Autodesk Inventor part; units mm, degrees
ref_plane "YZ Plane" through (0, 0, 0) normal (1, 0, 0) x (0, 1, 0)
ref_plane "XZ Plane" through (0, 0, 0) normal (0, 1, 0) x (-1, 0, 0)
ref_plane "XY Plane" through (0, 0, 0) normal (0, 0, 1) x (1, 0, 0)
sketch "Sketch8" plane through (0, 0, 0) normal (0, 1, 0) x (-1, 0, 0)
  line L0 (37.5, 50) -> (-37.5, 50)
  line L1 (-37.5, 50) -> (-37.5, -50)
  line L2 (-37.5, -50) -> (37.5, -50)
  line L3 (37.5, -50) -> (37.5, 50)
  point P0 (0, 0)
  point P1 (37.5, 0)
  point P2 (0, 50)
  dimension "d42" = 100
  dimension "d43" = 75
extrude "Extrusion5" add sketch "Sketch8" along normal blind 12
sketch "Sketch9" plane through (0, 12, 0) normal (0, 1, 0) x (1, 0, 0)
  line L0 (-37.5, 50) -> (-37.5, -50)
  line L1 (-37.5, -50) -> (37.5, -50)
  point P0 (0, 0)
  point P1 (-33.5, -46)
  point P2 (-33.5, 36)
  point P3 (33.5, 36)
  point P4 (33.5, -46)
  dimension "d46" = 67
  dimension "d47" = 82
  dimension "d48" = 4
  dimension "d49" = 4
hole "Hole3" at (-33.5, 12, 46) at (-33.5, 12, -36) at (33.5, 12, -36) at (33.5, 12, 46) direction (0, -1, 0) diameter 3.2 end through all
sketch "Sketch10" plane through (0, 12, 0) normal (0, 1, 0) x (1, 0, 0)
  line L0 (37.5, 50) -> (-37.5, 50)
  point P0 (0, 0)
  point P1 (-31, -36)
  point P2 (-31, 46)
  point P3 (31, 46)
  point P4 (31, -36)
  dimension "d57" = 62
  dimension "d58" = 82
  dimension "d59" = 4
  dimension "d60" = 31
hole "Hole4" at (-31, 12, 36) at (-31, 12, -46) at (31, 12, -46) at (31, 12, 36) direction (0, -1, 0) diameter 3.2 end through all
sketch "Sketch11" plane through (37.5, 0, 50) normal (1, 0, 0) x (0, 0, -1)
  line L0 (10, 8.5) -> (80, 8.5)
  line L1 (80, 8.5) -> (80, 0)
  line L2 (80, 0) -> (10, 0)
  line L3 (10, 0) -> (10, 8.5)
  line L4 (0, 0) -> (0, 12)
  line L5 (0, 0) -> (100, 0)
  point P0 (50, 0)
  point P1 (45, 0)
  dimension "d69" = 8.5
  dimension "d70" = 70
  dimension "d71" = 45
extrude "Extrusion6" cut sketch "Sketch11" against normal through all
sketch "Sketch12" plane through (-37.5, 0, 50) normal (0, 0, 1) x (1, 0, 0)
  line L0 (6.5, 8.5) -> (68.5, 8.5)
  line L1 (68.5, 8.5) -> (68.5, 0)
  line L2 (68.5, 0) -> (6.5, 0)
  line L3 (6.5, 0) -> (6.5, 8.5)
  line L4 (0, 0) -> (75, 0)
  point P0 (37.5, 0)
  point P1 (37.5, 0)
  dimension "d74" = 8.5
  dimension "d75" = 62
extrude "Extrusion7" cut sketch "Sketch12" against normal through all
sketch "Sketch13" plane through (37.5, 0, -50) normal (1, 0, 0) x (0, 0, -1)
  line L0 (0, 0) -> (0, 12)
  line L1 (0, 0) -> (-10, 0)
  line L2 (-10, 0) -> (-10, 8.5)
  line L3 (-10, 8.5) -> (0, 8.5)
  line L4 (0, 8.5) -> (0, 0)
  line L5 (-20, 8.5) -> (-20, 0)
  line L6 (-90, 8.5) -> (-20, 8.5)
  point P0 (-50, 0)
  dimension "d78" = 10
extrude "Extrusion8" cut sketch "Sketch13" against normal through all
fillet "Fillet1" radius 4 6 edges at (-37.5, 4.25, -40) (-37.5, 10.25, -50) (-37.5, 6, 50) (37.5, 6, 50) (37.5, 4.25, -40) (37.5, 10.25, -50)
sketch "Sketch14" plane through (0, 12, 0) normal (0, 1, 0) x (1, 0, 0)
  line L0 (-23.5, -44) -> (23.5, -44)
  line L1 (27.5, -40) -> (27.5, 40)
  line L2 (23.5, 44) -> (-23.5, 44)
  line L3 (-27.5, 40) -> (-27.5, -40)
  line L4 (-33.5, -50) -> (33.5, -50)
  line L5 (33.5, 50) -> (-33.5, 50)
  line L6 (-37.5, 46) -> (-37.5, -46)
  line L7 (37.5, -46) -> (37.5, 46)
  arc A0 (-27.5, -40) -> (-23.5, -44) centre (-23.5, -40) ccw
  arc A1 (23.5, -44) -> (27.5, -40) centre (23.5, -40) ccw
  arc A2 (27.5, 40) -> (23.5, 44) centre (23.5, 40) ccw
  arc A3 (-23.5, 44) -> (-27.5, 40) centre (-23.5, 40) ccw
  point P0 (0, 0)
  dimension "d82" = 6
  dimension "d83" = 6
  dimension "d84" = 10
  dimension "d85" = 10
  dimension "d86" = 4
extrude "Extrusion9" cut sketch "Sketch14" against normal through all
sketch "Sketch15" plane through (0, 12, 0) normal (0, 1, 0) x (1, 0, 0)
  circle A0 centre (-31, 46) radius 1.6
  circle A1 centre (-31, 46) radius 3
  circle A2 centre (-31, -36) radius 1.6
  circle A3 centre (-31, -36) radius 3
  circle A4 centre (31, -36) radius 1.6
  circle A5 centre (31, -36) radius 3
  circle A6 centre (31, 46) radius 1.6
  circle A7 centre (31, 46) radius 3
  point P0 (0, 0)
  dimension "d89" = 6
  dimension "d90" = 6
  dimension "d91" = 6
  dimension "d92" = 6
extrude "Extrusion10" add sketch "Sketch15" along normal blind 5
sketch "Sketch16" plane through (37.5, 8.5, -30) normal (0, -1, 0) x (1, 0, 0)
  circle A0 centre (-6.5, 66) radius 1.6
  circle A1 centre (-6.5, 66) radius 3
  line L0 (-6.5, 63) -> (-9.0981, 64.5)
  line L1 (-9.0981, 64.5) -> (-9.0981, 67.5)
  line L2 (-9.0981, 67.5) -> (-6.5, 69)
  line L3 (-6.5, 69) -> (-3.9019, 67.5)
  line L4 (-3.9019, 67.5) -> (-3.9019, 64.5)
  line L5 (-3.9019, 64.5) -> (-6.5, 63)
  circle A2 centre (-68.5, -16) radius 1.6
  circle A3 centre (-68.5, -16) radius 3
  line L6 (-68.5, -13) -> (-65.9019, -14.5)
  line L7 (-65.9019, -14.5) -> (-65.9019, -17.5)
  line L8 (-65.9019, -17.5) -> (-68.5, -19)
  line L9 (-68.5, -19) -> (-71.0981, -17.5)
  line L10 (-71.0981, -17.5) -> (-71.0981, -14.5)
  line L11 (-71.0981, -14.5) -> (-68.5, -13)
  circle A4 centre (-68.5, 66) radius 1.6
  circle A5 centre (-68.5, 66) radius 3
  line L12 (-68.5, 63) -> (-71.0981, 64.5)
  line L13 (-71.0981, 64.5) -> (-71.0981, 67.5)
  line L14 (-71.0981, 67.5) -> (-68.5, 69)
  line L15 (-68.5, 69) -> (-65.9019, 67.5)
  line L16 (-65.9019, 67.5) -> (-65.9019, 64.5)
  line L17 (-65.9019, 64.5) -> (-68.5, 63)
  circle A6 centre (-6.5, -16) radius 3
  line L18 (-6.5, -19) -> (-9.0981, -17.5)
  line L19 (-9.0981, -17.5) -> (-9.0981, -14.5)
  line L20 (-9.0981, -14.5) -> (-6.5, -13)
  line L21 (-6.5, -13) -> (-3.9019, -14.5)
  line L22 (-3.9019, -14.5) -> (-3.9019, -17.5)
  line L23 (-3.9019, -17.5) -> (-6.5, -19)
  point P0 (-37.5, 30)
  point P1 (-6.5, -16)
extrude "Extrusion11" cut sketch "Sketch16" against normal blind 3 contours L4 L5 L0 L1 L2 L3 | L7 L8 L9 L10 L11 L6 | A4 | L16 L17 L12 L13 L14 L15 | L22 L23 L18 L19 L20 L21
equation "\"d83\" = d82"
equation "\"d85\" = d84"
equation "\"d90\" = d89"
equation "\"d91\" = d89"
equation "\"d92\" = d89"
properties part number "phone_clamp_v2"
Input: part model. Units: mm. Frame: model coordinates. A direction names the side the tool comes from. Give positions to 0.01 mm unless a question says otherwise; leave off trailing zeros. Order: outer loops, then holes, each group sorted by start corner. A loop starts at its lowest first (then second) coordinate and runs counter-clockwise, first axis right, second up. Notation, with made-up numbers: (72, 10.25) - (111, 10.25) arc R21 cw to (111, 27.25) - close; hole circle Ø7 at (-5, 51.5). An arc over 180 degrees is marked (long way). Answer as a JSON object with one key per item and string values. Group by question number.
Q1. Cut plane D-D, the plane y = 4. Output: boundary loops of the cut face in (x, z), then the cut area to 3 significant figures.
Q2. Line query: probe 1 along X at (y, z) = (12.8, 36); probe 2 along Z at (x, y) = (33.5, 3.5); probe 3 along Z at (x, y) = (31, 14.2). Output: solid intervals per line, ascending.
Q3. First-contact query: pin 1 Ø3 at (x, y) = (-33.5, 4.5) entering from -Z; pin 2 Ø4 at (x, z) = (33.5, -36) entering from -Y; pin 3 Ø3.5 at (x, z) = (-33.5, 46) entering from +Y; pin 4 Ø1.9 at (x, z) = (31, 36) entering from -Y. Flat tips, straight axial feed; report the tip coordinate or a pass-through.
Q4. Cut plane C-C, the plane x = -12. Output: boundary loops of the cut face in (y, z).
Q5. Set-up query: faces 4 (the face through (-28.402, 10, 36)), 5 (the face through (34, 4, 40)), 6 (the face through (-32, 4, -40)), 7 (the face through (28, 12, -3)). Return all of +Z, -Z, +X, -X, +Y, -Y with unobstructed straight access to the full face (end or side cutting, diameter ignored); none if empty.
Q6. Cut plane B-B, the plane z = 23. Output: boundary loops of the cut face in (x, y).
Q7. Cut plane A-A, the plane y = 14.75. Output: boundary loops of the cut face in (x, z).
Q8. Mould query, pull axis X, two halves, no side actions, for faces 1 (the face through (34, 4, -30)), 2 (the face through (36.359, 4.31, -38.797)), 3 (the face through (0, 10, 44)). Classes: pulls with the +X half, pulls with the -X half, needs draft (parallel to the pull), parting line crosses it, or undercut.
Results:
{
 "1": {"outline": "(-37.5, -36) arc R4 ccw to (-33.5, -40) - (-31, -40) - (-31, -30) - (-37.5, -30) - close; (-37.5, 40) - (-31, 40) - (-31, 50) - (-33.5, 50) arc R4 ccw to (-37.5, 46) - close; (31, -40) - (33.5, -40) arc R4 ccw to (37.5, -36) - (37.5, -30) - (31, -30) - close; (31, 40) - (37.5, 40) - (37.5, 46) arc R4 ccw to (33.5, 50) - (31, 50) - close; hole circle Ø3.2 at (-33.5, -36); hole circle Ø3.2 at (-33.5, 46); hole circle Ø3.2 at (33.5, -36); hole circle Ø3.2 at (33.5, 46)", "area": "214 mm^2"},
 "2": {"probe 1": "-34 to -32.6, -29.4 to -28, 28 to 29.4, 32.6 to 34", "probe 2": "-40 to -37.6, -34.4 to -30, 40 to 44.4, 47.6 to 50", "probe 3": "-49 to -47.6, -44.4 to -43, 33 to 34.4, 37.6 to 39"},
 "3": {"pin 1": "z = -40", "pin 2": "y = 0", "pin 3": "y = 12", "pin 4": "through"},
 "4": {"outline": "(8.5, -50) - (12, -50) - (12, -44) - (8.5, -44) - close; (8.5, 44) - (12, 44) - (12, 50) - (8.5, 50) - close"},
 "5": {"face 4": "-Y", "face 5": "+X, -X, -Y", "face 6": "-Z, +X, -X, -Y", "face 7": "+Y"},
 "6": {"outline": "(-37.5, 8.5) - (-27.5, 8.5) - (-27.5, 12) - (-37.5, 12) - close; (27.5, 8.5) - (37.5, 8.5) - (37.5, 12) - (27.5, 12) - close"},
 "7": {"outline": "circle Ø6 at (-31, -46); circle Ø6 at (-31, 36); circle Ø6 at (31, -46); circle Ø6 at (31, 36); hole circle Ø3.2 at (-31, -46); hole circle Ø3.2 at (-31, 36); hole circle Ø3.2 at (31, -46); hole circle Ø3.2 at (31, 36)"},
 "8": {"face 1": "needs draft", "face 2": "pulls with the +X half", "face 3": "undercut"}
}
